Could you check a few things on this model? Use its own coordinates, in mm. Coordinates: 2 decimals unless noted, no trailing zeros. Write each loop counter-clockwise with the first axis right and the second up, starting at its lowest first coordinate (ties: lowest second). Pieces come first, ordered by that corner, then holes. Notation, with made-up numbers: M 34.25,69.25 L 78.25,69.25 A18 ccw 78.25,94.25 Z; hole C 0.5,27.5 d8. An arc over 180 degrees is marked long. Write item = value, one per line.
```python
from build123d import *

# Parameters (mm, degrees)
SKETCH1_R                = 32.5
BOSS_EXTRUDE1_DEPTH      = 392.5
FILLET1_R                = 5
SKETCH2_R                = 42.5
BOSS_EXTRUDE2_DEPTH      = 30
SKETCH3_R                = 20
CUT_EXTRUDE1_DEPTH       = 810
SKETCH4_R                = 30
SKETCH4_R_2              = 15
BOSS_EXTRUDE3_DEPTH      = 40
BOSS_EXTRUDE4_REACH      = 819.213
BOSS_EXTRUDE4_END_RADIUS = 30
SKETCH5_R                = 15
FILLET2_R                = 1


with BuildPart() as part:
    # Sketch1 → Boss-Extrude1 (new, symmetric)
    with BuildSketch(Plane(origin=(0, 0, 0), x_dir=(1, 0, 0), z_dir=(0, 1, 0))):
        with Locations(Location((0, 0, 0), (0, 0, 270))):
            Circle(SKETCH1_R)
    extrude(amount=BOSS_EXTRUDE1_DEPTH, both=True)

    # Fillet1
    fillet1_edges = [part.edges().sort_by_distance(p)[0] for p in [
        (0, 392.5, -32.5),
    ]]
    fillet(fillet1_edges, radius=FILLET1_R)

    # Sketch2 → Boss-Extrude2 (add)
    with BuildSketch(Plane.XZ.offset(392.5)):
        with Locations(Location((0, 0, 0), (0, 0, 270))):
            Circle(SKETCH2_R)
    extrude(amount=BOSS_EXTRUDE2_DEPTH)

    # Sketch3 → Cut-Extrude1 (cut)
    with BuildSketch(Plane.XZ.offset(422.5)):
        with Locations(Location((0, 0, 0), (0, 0, 270))):
            Circle(SKETCH3_R)
    extrude(amount=-CUT_EXTRUDE1_DEPTH, mode=Mode.SUBTRACT)



with BuildPart() as body_2:
    # Sketch4 → Boss-Extrude3 (new, symmetric)
    with BuildSketch(Plane.XY):
        with Locations((0, 487.5)):
            Circle(SKETCH4_R)
        with Locations((0, 487.5)):
            Circle(SKETCH4_R_2, mode=Mode.SUBTRACT)
    extrude(amount=BOSS_EXTRUDE3_DEPTH, both=True)


with BuildPart() as part_1:
    add(part.part)

    add(body_2.part)  # Boss-Extrude4 merges body 2
    # Boss-Extrude4: up to this cylinder (the profile starts outside it)
    boss_extrude4_end = Plane(origin=(0, 487.5, 0), z_dir=(0, 0, -1)) * Cylinder(BOSS_EXTRUDE4_END_RADIUS, 1699.426, mode=Mode.PRIVATE)
    # Sketch5 → Boss-Extrude4 (add, up to the surface)
    with BuildSketch(Plane(origin=(0, 392.5, 0), x_dir=(1, 0, 0), z_dir=(0, 1, 0)), mode=Mode.PRIVATE) as boss_extrude4_sk1:
        with Locations(Location((0, 0, 0), (0, 0, 90))):
            Circle(SKETCH5_R)
    boss_extrude4_tool1 = extrude(boss_extrude4_sk1.sketch, amount=BOSS_EXTRUDE4_REACH, mode=Mode.PRIVATE) - boss_extrude4_end
    add(boss_extrude4_tool1.solids().sort_by_distance((0, 392.5, 0))[0])

    # Fillet2
    fillet2_edges = [part_1.edges().sort_by_distance(p)[0] for p in [
        (0, -392.5, 42.5),
        (0, -422.5, 42.5),
    ]]
    fillet(fillet2_edges, radius=FILLET2_R)


solid = part_1.part
```
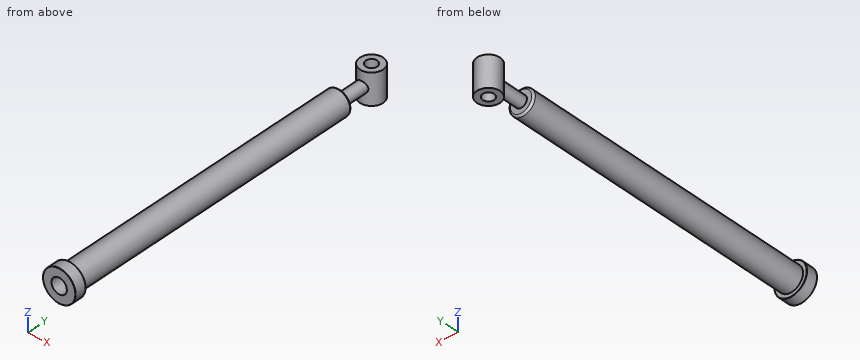
Item 1: Imagine slicing it at D-D (y = 360). Write out the boundary of the cut face in (x, z), and give its area (3 significant figures).
Numbers:
outline = C 0,0 d65; hole C 0,0 d40
area = 2,060 mm²
Item 2: Imagine slicing it at C-C (z = 0). Write out the boundary of the cut face in (x, y), and give its area (3 significant figures).
Numbers:
outline = M -42.5,-421.5 A1 ccw -41.5,-422.5 L -20,-422.5 L -20,387.5 L 20,387.5 L 20,-422.5 L 41.5,-422.5 A1 ccw 42.5,-421.5 L 42.5,-393.5 A1 ccw 41.5,-392.5 L 32.5,-392.5 L 32.5,387.5 A5 ccw 27.5,392.5 L 15,392.5 L 15,461.52 A30 ccw long -15,461.52 L -15,392.5 L -27.5,392.5 A5 ccw -32.5,387.5 L -32.5,-392.5 L -41.5,-392.5 A1 ccw -42.5,-393.5 Z; hole C 0,487.5 d30
area = 25,300 mm²
Item 3: If I drill on line 1 along X through (y, z) = (487, -14); line 2 along Y through (x, z) = (0, -5.5); line 3 along X through (y, z) = (-146, 0), over which ranges is the centre line in solid material (lowest first)?
Numbers:
line_1 = -30 to -14.99, 14.99 to 30
line_2 = 387.5 to 472.5, 502.5 to 517.5
line_3 = -32.5 to -20, 20 to 32.5
Item 4: Imagine slicing it at A-A (y = 487.5). Write out the boundary of the cut face in (x, z), and give its area (3 significant figures).
Numbers:
outline = M -30,-40 L -15,-40 L -15,40 L -30,40 Z; M 15,-40 L 30,-40 L 30,40 L 15,40 Z
area = 2,400 mm²
Item 5: I'm going to push flat-ended pins straight in: P1, Ø4, axis at y = 264.5, z = 17, coming from the +X side; P2, Ø3, axis at x = -7.5, z = -5.5, coming from the -Y side; P3, Ø18, axis at x = 3, y = 495, coming from the -Z side; P4, Ø24, axis at x = 0, y = 487.5, coming from the +Z side. Where does each tip first touch, or does it pass through?
Numbers:
P1 = 28.83
P2 = 387.5
P3 = -40
P4 = through
